Build history of the part. All positions in model axes, mm. Give positions to 0.01 mm unless a question says otherwise; leave off trailing zeros. Order: outer loops, then holes, each group sorted by start corner. A loop starts at its lowest first (then second) coordinate and runs counter-clockwise, first axis right, second up. Notation, with made-up numbers: (38, -18.5) - (81, -18.5) arc R24 cw to (81, 17.5) - close; hole circle Ø1 at (43, 49). An arc over 180 degrees is marked (long way). One line per item, written item: value.
```python
from build123d import *

# Parameters (mm, degrees)
F0_W      = 101.6
F0_H      = 76.2
F1_DEPTH  = 50.8
F1_FACE_W = 101.6
F1_FACE_H = 76.2
F2_DEPTH  = 38.1
F3_R      = 26.108539
F4_DEPTH  = 101.6


with BuildPart() as f1:
    # F0 (on Front) → F1 (new body)
    with BuildSketch(Plane.XZ):
        with Locations((50.8, 38.1)):
            Rectangle(F0_W, F0_H)
    extrude(amount=-F1_DEPTH)

    # F1_face (on face) → F2 (join)
    with BuildSketch(Plane(origin=(50.8, 0, 38.1), x_dir=(1, 0, 0), z_dir=(0, -1, 0))):
        Rectangle(F1_FACE_W, F1_FACE_H)
    extrude(amount=F2_DEPTH)

    # F3 (on face) → F4 (cut)
    with BuildSketch(Plane.YZ.offset(101.6)):
        with Locations((8.532524, 37.164632)):
            Circle(F3_R)
    extrude(amount=-F4_DEPTH, mode=Mode.SUBTRACT)


solid = f1.part
```
(1) Pin check, flat tip, straight feed: P1, Ø5, axis at y = -26, z = 53, coming from the -X side. Stop position of the tip, or through.
Completed:
P1: x = 0
(2) Slice it at B-B, the plane y = 24. Give the cut face in (x, z), and give its area (3 significant figures).
Completed:
outline: (0, 0) - (101.6, 0) - (101.6, 16.13) - (0, 16.13) - close; (0, 58.2) - (101.6, 58.2) - (101.6, 76.2) - (0, 76.2) - close
area: 3,470 mm²
(3) Drill centre lines: line 1 (Z direction, x = 6.5, y = -7); line 2 (Z direction, x = 75.5, y = -12.5); line 3 (Y direction, x = 92, z = 43). Where is each one in solid material? Low to high.
Completed:
line 1: 0 to 16.18, 58.15 to 76.2
line 2: 0 to 21.7, 52.63 to 76.2
line 3: -38.1 to -16.92, 33.98 to 50.8
(4) Pull direction Y, two halves, no side cores. Call faces 1 (the face through (50, -38.1, 39)), 2 (the face through (51.51, 22.57, 59.18)), 3 (the face through (50, 7, 0)), 4 (the face through (50, 50.8, 39)): +Y half, -Y half, draft (parallel to the pull), parting line (faces both ways), or undercut.
Completed:
face 1: -Y half
face 2: undercut
face 3: draft
face 4: +Y half
(5) Slice it at A-A, the plane z = 34.5. Give the cut face in (x, y).
Completed:
outline: (0, -38.1) - (101.6, -38.1) - (101.6, -17.44) - (0, -17.44) - close; (0, 34.5) - (101.6, 34.5) - (101.6, 50.8) - (0, 50.8) - close
(6) Slice it at C-C, the plane x = 12.5. Give the cut face in (y, z), and give its area (3 significant figures).
Completed:
outline: (-38.1, 0) - (50.8, 0) - (50.8, 76.2) - (-38.1, 76.2) - close; hole circle Ø52.22 at (8.53, 37.16)
area: 4,630 mm²
